Verification items for the finished model (mm, model axes). Face numbers are marked on the shaded views. A direction names the side the tool comes from. Give positions to 0.01 mm unless a question says otherwise; leave off trailing zeros. Order: outer loops, then holes, each group sorted by start corner. A loop starts at its lowest first (then second) coordinate and runs counter-clockwise, first axis right, second up.
(1) Mould release check, pull along X, two halves, no side actions. Record for the marked faces 3 and 4: pulls with the +X half, pulls with the -X half, needs draft (parallel to the pull), parting line crosses it, or undercut.
(2) Sectioned sample at B-B on x = -21.6. Record the cut outline in (y, z).
(3) Sectioned sample at A-A on y = -33. Record the cut outline in (x, z), plus the area to 3 significant figures.
(4) Sectioned sample at D-D on x = 14. Record the cut outline in (y, z).
(5) Gauge pin test, flat ends, axial feed: pin 1 (0.7 mm diameter, centred on x = -3, y = 38, fed in from -Z); pin 2 (3 mm diameter, centred on x = 19.5, z = 0.5, fed in from -Y); pin 3 (10 mm diameter, centred on x = 20, y = -2.5, fed in from +Z). Record the tip position at first contact, or that the pin passes through.
(6) Sectioned sample at C-C on x = 0. Record the cut outline in (y, z), plus the area to 3 significant figures.
(7) Access from +Z, -Z, +X, -X, +Y, -Y to the whole of each face (thin tool, end or side, straight path). Record for the marked faces 1 and 2.
(8) Scan lines: L1, parallel to Y at x = -21.6, z = 1; L2, parallel to Z at x = -8, y = 20; L3, parallel to X at y = -41.5, z = 3.75. Record each from-to range of solid material in increasing order.
```python
from build123d import *

# Parameters (mm, degrees)
F0_R          = 1.5875
F0_W          = 4.5
F0_H          = 2
F3_DEPTH      = 1.5
F4_START      = 36.85
F1_R          = 3.15
F4_DEPTH      = 9.6
F5_START      = -32.95
F2_W          = 12.9
F2_H          = 2.5
F5_DEPTH      = 5.3
F0_H_2        = 1
F6_DEPTH      = 2.75
F6_DEPTH_BACK = 0.75


with BuildPart() as f3:
    # F0 (on Top) → F3 (new body)
    with BuildSketch(Plane.XY):
        Polygon((-25.4, -36.85), (25.4, -36.85), (25.4, 36.85), (-10.15, 36.85), (-10.15, 34.85), (-14.65, 34.85), (-14.65, 36.85), (-25.4, 36.85), align=None)
        with Locations((-21.6, -33)):
            Circle(F0_R, mode=Mode.SUBTRACT)
        with Locations((21.6, -33)):
            Circle(F0_R, mode=Mode.SUBTRACT)
        with Locations((-21.6, 33)):
            Circle(F0_R, mode=Mode.SUBTRACT)
        with Locations((21.6, 33)):
            Circle(F0_R, mode=Mode.SUBTRACT)
        with Locations((-12.4, 35.85)):
            Rectangle(F0_W, F0_H)
    extrude(amount=F3_DEPTH)

    # F1 (on Front) → F4 (join)
    with BuildSketch(Plane.XZ.offset(F4_START)):
        with Locations((-14, 1.7)):
            Circle(F1_R)
        with Locations((0, 1.7)):
            Circle(F1_R)
        with Locations((14, 1.7)):
            Circle(F1_R)
    extrude(amount=F4_DEPTH)

    # F2 (on Front) → F5 (join)
    with BuildSketch(Plane.XZ.offset(F5_START)):
        with Locations((0, 2.75)):
            Rectangle(F2_W, F2_H)
    extrude(amount=-F5_DEPTH)

    # F0 (on Top) → F6 (join, two sides)
    with BuildSketch(Plane.XY) as f6_sk:
        with Locations((-12.4, 35.85)):
            Rectangle(F0_W, F0_H)
        with Locations((-12.4, 37.35)):
            Rectangle(F0_W, F0_H_2)
    extrude(amount=F6_DEPTH)
    extrude(f6_sk.sketch, amount=-F6_DEPTH_BACK)


solid = f3.part
```
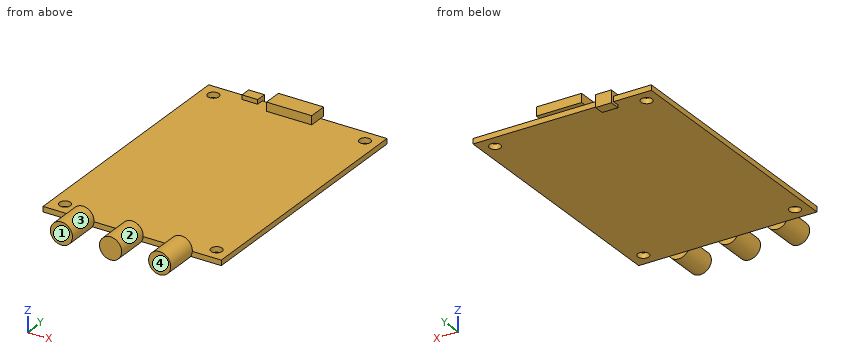
Ans:
1. face 3: undercut
1. face 4: needs draft
2. outline: (-36.85, 0) - (-34.59, 0) - (-34.59, 1.5) - (-36.85, 1.5) - close; (-31.41, 0) - (31.41, 0) - (31.41, 1.5) - (-31.41, 1.5) - close; (34.59, 0) - (36.85, 0) - (36.85, 1.5) - (34.59, 1.5) - close
3. outline: (-25.4, 0) - (-23.19, 0) - (-23.19, 1.5) - (-25.4, 1.5) - close; (-20.01, 0) - (20.01, 0) - (20.01, 1.5) - (-20.01, 1.5) - close; (23.19, 0) - (25.4, 0) - (25.4, 1.5) - (23.19, 1.5) - close
3. area: 66.7 mm2
4. outline: (-46.45, -1.45) - (-36.85, -1.45) - (-36.85, 0) - (36.85, 0) - (36.85, 1.5) - (-36.85, 1.5) - (-36.85, 4.85) - (-46.45, 4.85) - close
5. pin 1: stops at z = 1.5
5. pin 2: stops at y = -36.85
5. pin 3: stops at z = 1.5
6. outline: (-46.45, -1.45) - (-36.85, -1.45) - (-36.85, 0) - (36.85, 0) - (36.85, 1.5) - (38.25, 1.5) - (38.25, 4) - (32.95, 4) - (32.95, 1.5) - (-36.85, 1.5) - (-36.85, 4.85) - (-46.45, 4.85) - close
6. area: 184 mm2
7. face 1: +Z, -Z, +X, -X, -Y
7. face 2: -Y
8. L1: y = -36.85 to -34.59, -31.41 to 31.41, 34.59 to 36.85
8. L2: z = 0 to 1.5
8. L3: x = -16.39 to -11.61, -2.39 to 2.39, 11.61 to 16.39
